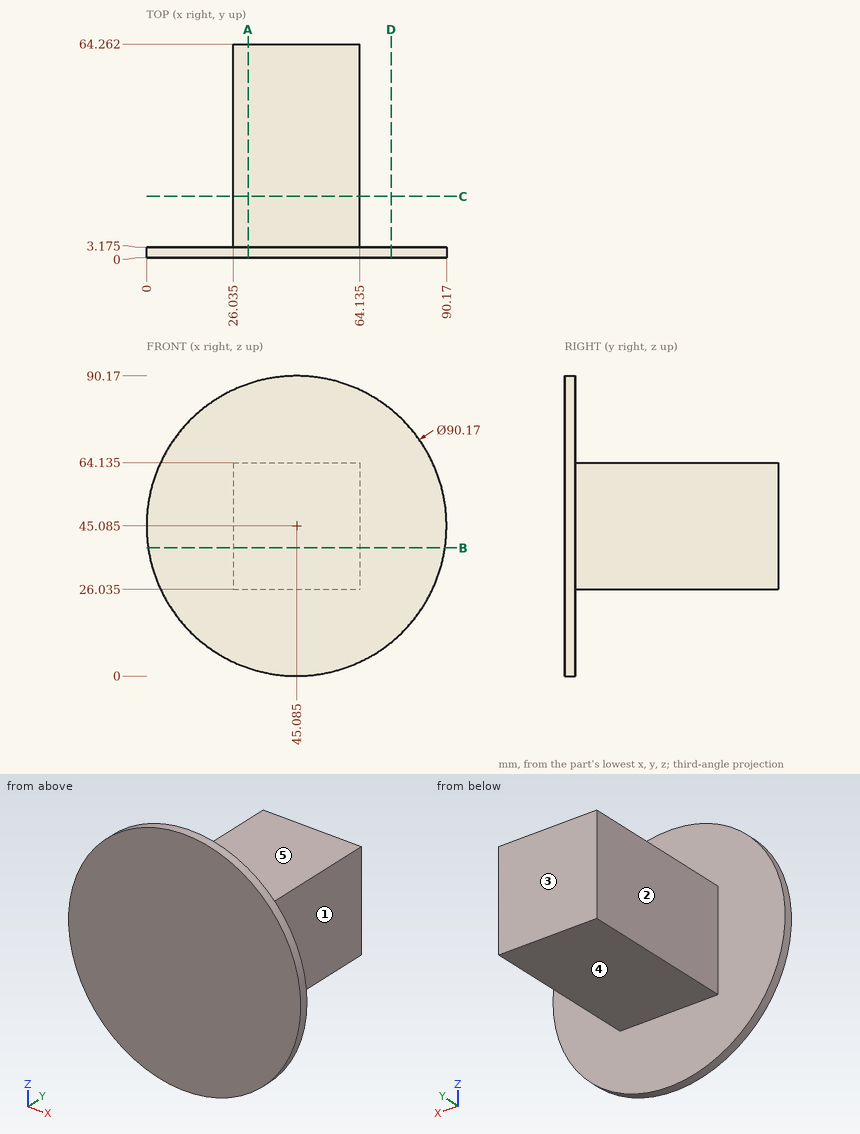
Study the drawing (mm; zero at the part's minimum x, y, z) and answer. A direction names the side the tool comes from. Coordinates: 2 decimals unless noted, no trailing zeros. Write each loop counter-clockwise with the first axis right and the second up, starting at its lowest first coordinate (ties: lowest second). Pieces come first, ordered by that corner, then holes. Notation, with made-up numbers: M 76.5,19 L 114.5,19 A8 ccw 114.5,34 Z; hole C -14.5,69 d10. An arc over 180 degrees is marked long. Use a Markdown table: item, result. Add a question column.
1. Section A-A (x = 30.5) is taken. Give the vertices of the cut face in (y, z) (3 decimals).
2. Which of the six approach directions +Z, -Z, +X, -X, +Y, -Y give full straight-line access (tool end or side, diameter ignored) to the marked faces 1, 2, 3, 4 and 5?
3. Given P1, Ø5, axis at x = 12, z = 73.5, coming from the +Y side (3 decimals); P2, Ø5, axis at y = 33, z = 35, coming from the +X side (3 decimals); P3, Ø1, axis at x = 18.5, z = 66, coming from the -Y side; P4, Ø11.5, axis at x = 43.5, y = 23.5, coming from the -Z side (3 decimals), each flat-ended and moving along its own axis, determine where each tip first touches the part or whether it passes through.
4. Section C-C (y = 18.5) is taken. Give the vertices of the cut face in (x, z) (3 decimals), plus the area to 3 significant figures.
5. Straight lines are drawn through the part: line 1 along X through (y, z) = (61.5, 35) (3 decimals); line 2 along Y through (x, z) = (20.5, 72.5) (3 decimals). For each, find the intervals that lie inside material, in ascending order. Write a range as [from, to].
6. Section D-D (x = 73.5) is taken. Give the vertices of the cut face in (y, z) (1 decimal).
7. Section B-B (z = 38.5) is taken. Give the vertices of the cut face in (x, y) (3 decimals), plus the area to 3 significant figures.
Data:
| question | item | result |
|---|---|---|
| 1 | outline | M 0,2.424 L 3.175,2.424 L 3.175,26.035 L 64.262,26.035 L 64.262,64.135 L 3.175,64.135 L 3.175,87.746 L 0,87.746 Z |
| 2 | face 1 | +Z, -Z, +X, +Y |
| 2 | face 2 | +Z, -Z, -X, +Y |
| 2 | face 3 | +Z, -Z, +X, -X, +Y |
| 2 | face 4 | -Z, +X, -X, +Y |
| 2 | face 5 | +Z, +X, -X, +Y |
| 3 | P1 | stops at y = 3.175 |
| 3 | P2 | stops at x = 64.135 |
| 3 | P3 | stops at y = 0 |
| 3 | P4 | stops at z = 26.035 |
| 4 | outline | M 26.035,26.035 L 64.135,26.035 L 64.135,64.135 L 26.035,64.135 Z |
| 4 | area | 1,450 mm2 |
| 5 | line 1 | x = [26.035, 64.135] |
| 5 | line 2 | y = [0, 3.175] |
| 6 | outline | M 0,10.1 L 3.2,10.1 L 3.2,80.1 L 0,80.1 Z |
| 7 | outline | M 0.483,0 L 89.687,0 L 89.687,3.175 L 64.135,3.175 L 64.135,64.262 L 26.035,64.262 L 26.035,3.175 L 0.483,3.175 Z |
| 7 | area | 2,610 mm2 |
